The model under review builds one solid part; all positions refer to its coordinate system, in mm. A direction names the side the tool comes from. Round coordinates to 2 decimals unless told otherwise and drop trailing zeros. Order: outer loops, then holes, each group sorted by start corner. A loop starts at its lowest first (then second) coordinate and runs counter-clockwise, first axis right, second up. Notation, with made-up numbers: (22.5, 50.5) -> (32.5, 50.5) arc R37 ccw to (32.5, 87.5) -> close; hole circle Ø6 at (35.25, 20.5). An arc over 180 degrees is marked (long way). Return JSON: item names as keys, results as strings. Group by question number.
from build123d import *

# Parameters (mm, degrees)
SKETCH2_R           = 2
SKETCH2_R_2         = 3.455
SKETCH2_R_3         = 3
BOSS_EXTRUDE1_DEPTH = 6.35
SKETCH3_R           = 4
SKETCH3_R_2         = 2
BOSS_EXTRUDE2_DEPTH = 10


with BuildPart() as part:
    # Sketch2 → Boss-Extrude1 (new body)
    with BuildSketch(Plane(origin=(0, 0, 0), x_dir=(1, 0, 0), z_dir=(0, 1, 0))):
        Polygon((0, 0), (280, 0), (280, 374.8), (262.142723834, 401.006270851), (140, 401.01), (17.857276166, 401.006270851), (0, 374.8), align=None)
        with Locations((45.125976945, 35.709590933)):
            Circle(SKETCH2_R, mode=Mode.SUBTRACT)
        with Locations((45.125976945, 110.709590933)):
            Circle(SKETCH2_R, mode=Mode.SUBTRACT)
        with Locations((104.125976945, 35.709590933)):
            Circle(SKETCH2_R, mode=Mode.SUBTRACT)
        with Locations((104.125976945, 110.709590933)):
            Circle(SKETCH2_R, mode=Mode.SUBTRACT)
        with Locations((163.125976945, 35.709590933)):
            Circle(SKETCH2_R, mode=Mode.SUBTRACT)
        with Locations((163.125976945, 110.709590933)):
            Circle(SKETCH2_R, mode=Mode.SUBTRACT)
        with Locations((57.382352913, 171.377840784)):
            Circle(SKETCH2_R_2, mode=Mode.SUBTRACT)
        with Locations((132.032352913, 171.377840784)):
            Circle(SKETCH2_R_2, mode=Mode.SUBTRACT)
        with Locations((252.523722024, 10.5)):
            Circle(SKETCH2_R, mode=Mode.SUBTRACT)
        with Locations((218.233722024, 28.5)):
            Circle(SKETCH2_R, mode=Mode.SUBTRACT)
        with Locations((183.943722024, 10.5)):
            Circle(SKETCH2_R, mode=Mode.SUBTRACT)
        with Locations((265, 88.605509424)):
            Circle(SKETCH2_R_3, mode=Mode.SUBTRACT)
        with Locations((265, 58.605509424)):
            Circle(SKETCH2_R_3, mode=Mode.SUBTRACT)
        with Locations((15, 58.605509424)):
            Circle(SKETCH2_R_3, mode=Mode.SUBTRACT)
        with Locations((15, 88.605509424)):
            Circle(SKETCH2_R_3, mode=Mode.SUBTRACT)
        with Locations((265, 316.194490576)):
            Circle(SKETCH2_R_3, mode=Mode.SUBTRACT)
        with Locations((265, 286.194490576)):
            Circle(SKETCH2_R_3, mode=Mode.SUBTRACT)
        with Locations((15, 316.194490576)):
            Circle(SKETCH2_R_3, mode=Mode.SUBTRACT)
        with Locations((15, 286.194490576)):
            Circle(SKETCH2_R_3, mode=Mode.SUBTRACT)
    extrude(amount=BOSS_EXTRUDE1_DEPTH)

    # Sketch3 → Boss-Extrude2 (add)
    with BuildSketch(Plane(origin=(0, 6.35, 0), x_dir=(1, 0, 0), z_dir=(0, 1, 0))):
        with Locations((241.321633488, 94.932700401)):
            Circle(SKETCH3_R)
        with Locations((241.321633488, 94.932700401)):
            Circle(SKETCH3_R_2, mode=Mode.SUBTRACT)
        with Locations((198.776633488, 94.932700401)):
            Circle(SKETCH3_R)
        with Locations((198.776633488, 94.932700401)):
            Circle(SKETCH3_R_2, mode=Mode.SUBTRACT)
        with Locations((198.776633488, 141.287700401)):
            Circle(SKETCH3_R)
        with Locations((198.776633488, 141.287700401)):
            Circle(SKETCH3_R_2, mode=Mode.SUBTRACT)
        with Locations((241.321633488, 141.287700401)):
            Circle(SKETCH3_R)
        with Locations((241.321633488, 141.287700401)):
            Circle(SKETCH3_R_2, mode=Mode.SUBTRACT)
    extrude(amount=BOSS_EXTRUDE2_DEPTH)


solid = part.part
Item 1: Consider section A-A on y = 11.75. State the section outline as (x, z) points.
Item 2: The part is to be moulded in two halves that separate along Z. For faces 3 (the face through (239, 16.35, -140)), 4 (the face through (271.196, 3.131, -387.72)), 5 (the face through (202.47, 11.28, -93.4)), say which applies: +Z half, -Z half, draft (parallel to the pull), parting line (faces both ways), or undercut.
Item 3: Consider section B-B on z = -126. State the section outline as (x, y) points, plus the area to 3 significant figures.
Item 4: Consider section C-C on x = 36. State the section outline as (y, z) points.
Item 5: Wall thickness on line 1 along X through (y, z) = (1.5, -10.5); line 2 along Z through (x, y) = (232.5, 5.75); line 3 along Y through (x, z) = (228, -370): over which ranges is each line inside the solid? List them lowest first.
Item 6: For faces 1 (the face through (242, 16.35, -97)), 2 (the face through (245.017, 11.28, -93.401)), list the 3-axis set-ups (+Z, -Z, +X, -X, +Y, -Y) from which the entire face can be reached by the end or side of a thin tool; tool diameter is ignored.
Item 7: Insertion check: pin 1 Ø5 at (x, z) = (15, -88.61) entering from -Y; pin 2 Ø5 at (x, z) = (117, -157) entering from +Y; pin 3 Ø6 at (x, z) = (104.5, -358.5) entering from -Y; pin 4 Ø6 at (x, y) = (199, 14.5) entering from -Z. Each pin has a flat end and moves straight along its axis. Give the tip position at first contact, or say it passes through.
Values:
{
 "1": {"outline": "circle Ø8 at (198.78, -141.29); circle Ø8 at (198.78, -94.93); circle Ø8 at (241.32, -141.29); circle Ø8 at (241.32, -94.93); hole circle Ø4 at (198.78, -141.29); hole circle Ø4 at (198.78, -94.93); hole circle Ø4 at (241.32, -141.29); hole circle Ø4 at (241.32, -94.93)"},
 "2": {"face 3": "draft", "face 4": "-Z half", "face 5": "undercut"},
 "3": {"outline": "(0, 0) -> (280, 0) -> (280, 6.35) -> (0, 6.35) -> close", "area": "1,780 mm^2"},
 "4": {"outline": "(0, -401.01) -> (6.35, -401.01) -> (6.35, 0) -> (0, 0) -> close"},
 "5": {"line 1": "0 to 181.94, 185.94 to 250.52, 254.52 to 280", "line 2": "-401.01 to 0", "line 3": "0 to 6.35"},
 "6": {"face 1": "+Z, -Z, +X, -X, +Y", "face 2": "+Y"},
 "7": {"pin 1": "through", "pin 2": "y = 6.35", "pin 3": "y = 0", "pin 4": "z = -145.29"}
}
